Can you work these out from the model? Positions are in its coordinate system, mm. A direction names the side the tool comes from. Coordinates: 2 decimals unless noted, no trailing zeros. Order: outer loops, then holes, each group sorted by start corner. A loop starts at its lowest first (then second) coordinate and runs counter-clockwise, first axis right, second up. Notation, with made-up numbers: (-14, 57) -> (26, 57) arc R33 ccw to (26, 90) -> close; hole circle Ø4 at (-4, 14.25). An arc over 180 degrees is marked (long way). Answer as CSV lines item,"result".
from build123d import *

# Parameters (mm, degrees)
BODY_DEPTH = 12
PINS_SK2_W = 0.6
PINS_SK2_H = 0.6
PINS_DEPTH = 15.5
CAP_SK3_R  = 6
CAP_DEPTH  = 5.6


with BuildPart() as part:
    # Body_Sk1 → Body (new body)
    with BuildSketch(Plane(origin=(0, 28.4, 0), x_dir=(1, 0, 0), z_dir=(0, 1, 0))):
        with BuildLine():
            Line((30.3, 28.5), (41.7, 28.5))
            ThreePointArc((41.7, 28.5), (41.912132034, 28.412132034), (42, 28.2))
            Line((42, 28.2), (42, 16.8))
            ThreePointArc((42, 16.8), (41.912132034, 16.587867966), (41.7, 16.5))
            Line((41.7, 16.5), (30.3, 16.5))
            ThreePointArc((30.3, 16.5), (30.087867966, 16.587867966), (30, 16.8))
            Line((30, 16.8), (30, 28.2))
            ThreePointArc((30, 28.2), (30.087867966, 28.412132034), (30.3, 28.5))
        make_face()
    extrude(amount=-BODY_DEPTH)

    # Pins_Sk2 → Pins (add)
    with BuildSketch(Plane(origin=(0, 28.4, 0), x_dir=(1, 0, 0), z_dir=(0, 1, 0))):
        with Locations((31.5, 25)):
            Rectangle(PINS_SK2_W, PINS_SK2_H)
        with Locations((31.5, 20)):
            Rectangle(PINS_SK2_W, PINS_SK2_H)
        with Locations((36, 25)):
            Rectangle(PINS_SK2_W, PINS_SK2_H)
        with Locations((36, 20)):
            Rectangle(PINS_SK2_W, PINS_SK2_H)
        with Locations((40.5, 25)):
            Rectangle(PINS_SK2_W, PINS_SK2_H)
        with Locations((40.5, 20)):
            Rectangle(PINS_SK2_W, PINS_SK2_H)
    extrude(amount=-PINS_DEPTH)

    # Cap_Sk3 → Cap (add)
    with BuildSketch(Plane(origin=(0, 28.4, 0), x_dir=(1, 0, 0), z_dir=(0, 1, 0))):
        with Locations(Location((36, 22.5, 0), (0, 0, 270))):
            Circle(CAP_SK3_R)
    extrude(amount=CAP_DEPTH)


solid = part.part
Q1. Imagine slicing it at B-B (y = 32). List the corners of the cut face in (x, z) for me.
Solution:
outline,"circle Ø12 at (36, -22.5)"
Q2. Imagine slicing it at A-A (x = 40.5). List the corners of the cut face in (y, z) for me.
Solution:
outline,"(12.9, -25.3) -> (16.4, -25.3) -> (16.4, -28.5) -> (28.4, -28.5) -> (28.4, -26.47) -> (34, -26.47) -> (34, -18.53) -> (28.4, -18.53) -> (28.4, -16.5) -> (16.4, -16.5) -> (16.4, -19.7) -> (12.9, -19.7) -> (12.9, -20.3) -> (16.4, -20.3) -> (16.4, -24.7) -> (12.9, -24.7) -> close"
Q3. Imagine slicing it at D-D (x = 32.25). List the corners of the cut face in (y, z) for me, and give its area (3 significant figures).
Solution:
outline,"(16.4, -28.5) -> (28.4, -28.5) -> (28.4, -27.18) -> (34, -27.18) -> (34, -17.82) -> (28.4, -17.82) -> (28.4, -16.5) -> (16.4, -16.5) -> close"
area,"196 mm2"
Q4. Which directions (+Z, -Z, +X, -X, +Y, -Y) give clear straight access to the entire face, cutting with the end or side of a thin tool? Please do faces 1 (the flat face through (41, 28.4, -18)), 2 (the flat face through (31, 28.4, -18)), 3 (the flat face through (41, 28.4, -27)).
Solution:
face 1,"+Z, +X, +Y"
face 2,"+Z, -X, +Y"
face 3,"-Z, +X, +Y"
Q5. For P1, Ø5, axis at x = 32, y = 31.5, coming from the +Z side; P2, Ø0.7, axis at y = 14, z = -25, coming from the +X side; P3, Ø2, axis at x = 32.5, z = -23.5, coming from the -Y side, each with a flat end and sliding along its axis, tell me the tip position at first contact or that it passes through.
Solution:
P1,"z = -16.69"
P2,"x = 40.8"
P3,"y = 16.4"
Q6. Imagine slicing it at C-C (z = -23.5). List the corners of the cut face in (x, y) for me.
Solution:
outline,"(30, 16.4) -> (42, 16.4) -> (42, 28.4) -> (41.92, 28.4) -> (41.92, 34) -> (30.08, 34) -> (30.08, 28.4) -> (30, 28.4) -> close"
Q7. If I drill on line 1 (Z direction, x = 40.75, y = 16); line 2 (Y direction, x = 31, z = -18.75); line 3 (Y direction, x = 36.25, z = -25.5), over which ranges is the centre line in solid material (lowest first)?
Solution:
line 1,"-25.3 to -24.7, -20.3 to -19.7"
line 2,"16.4 to 28.4"
line 3,"16.4 to 34"
